Verification items for this drawing (mm, ordinates from the low corner). A direction names the side the tool comes from. Give positions to 0.01 mm unless a question says otherwise; leave off trailing zeros. Write each loop counter-clockwise with the first axis right and the second up, starting at its lowest first coordinate (ties: lowest second). Pieces come first, ordered by that corner, then holes. Notation, with made-up numbers: (36.25, -16.75) -> (65.25, -16.75) arc R21 ccw to (65.25, -11.75) -> close; hole circle Ø5 at (61, 25.5). An arc over 180 degrees is marked (long way). Answer as a JSON object with one key per item and string values.
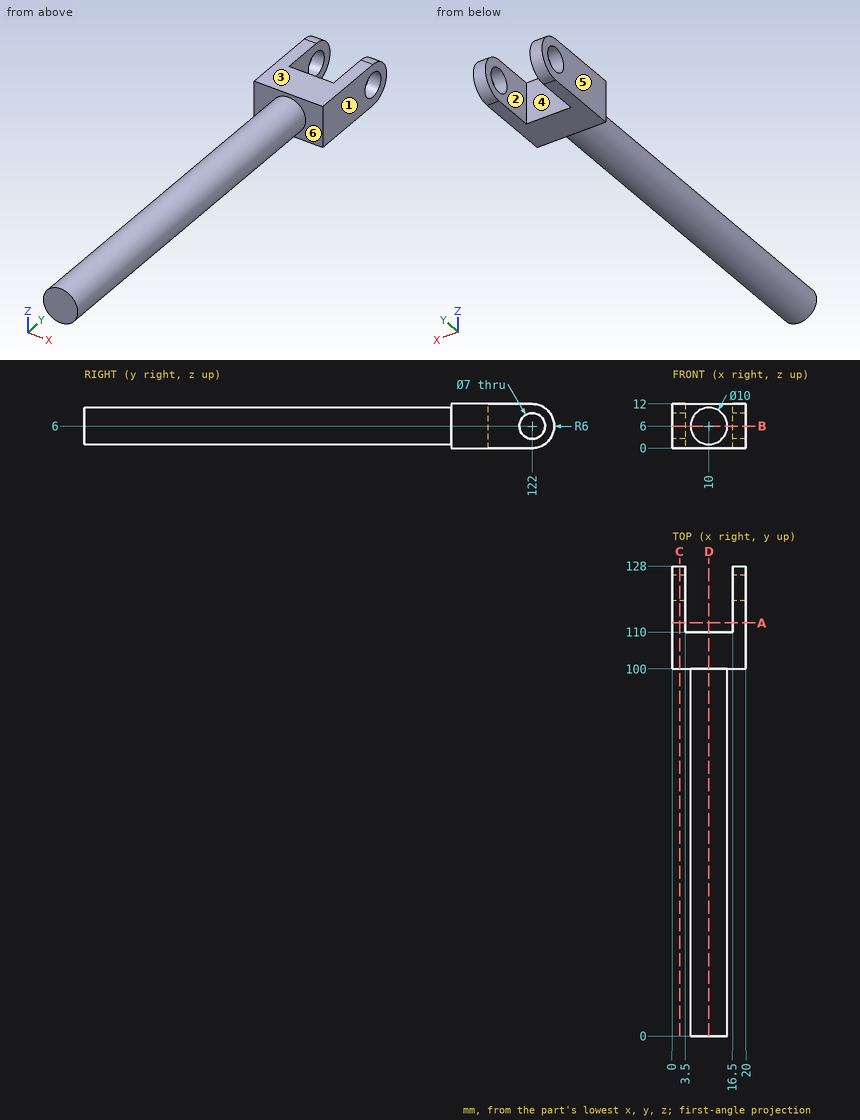
1. Sectioned sample at D-D, the plane x = 10. Enter the section's corners in (y, z).
Determined:
{"outline": "(0, 1) -> (100, 1) -> (100, 0) -> (110, 0) -> (110, 12) -> (100, 12) -> (100, 11) -> (0, 11) -> close"}
2. Scan lines: L1, parallel to Z at x = 18.6, y = 122; L2, parallel to Y at x = 1.85, z = 6; L3, parallel to X at y = 8, z = 6.25. Record each from-to range of solid material in increasing order. Write a range as [from, to].
Determined:
{"L1": "[0, 2.5], [9.5, 12]", "L2": "[100, 118.5], [125.5, 128]", "L3": "[5.01, 14.99]"}
3. Access from +Z, -Z, +X, -X, +Y, -Y to the whole of each face (thin tool, end or side, straight path). Record for the marked faces 4, 5 and 6.
Determined:
{"face 4": "+Z, -Z, +Y", "face 5": "+Z, -Z, -X, +Y, -Y", "face 6": "-Y"}
4. Sectioned sample at C-C, the plane x = 2. Enter the section's corners in (y, z).
Determined:
{"outline": "(100, 0) -> (122, 0) arc R6 ccw to (122, 12) -> (100, 12) -> close; hole circle Ø7 at (122, 6)"}
5. Sectioned sample at B-B, the plane z = 6. Enter the section's corners in (x, y), plus the area to 3 significant figures.
Determined:
{"outline": "(0, 100) -> (5, 100) -> (5, 0) -> (15, 0) -> (15, 100) -> (20, 100) -> (20, 118.5) -> (16.5, 118.5) -> (16.5, 110) -> (3.5, 110) -> (3.5, 118.5) -> (0, 118.5) -> close; (0, 125.5) -> (3.5, 125.5) -> (3.5, 128) -> (0, 128) -> close; (16.5, 125.5) -> (20, 125.5) -> (20, 128) -> (16.5, 128) -> close", "area": "1,280 mm^2"}
6. Sectioned sample at A-A, the plane y = 112.5. Enter the section's corners in (x, z), plus the area to 3 significant figures.
Determined:
{"outline": "(0, 0) -> (3.5, 0) -> (3.5, 12) -> (0, 12) -> close; (16.5, 0) -> (20, 0) -> (20, 12) -> (16.5, 12) -> close", "area": "84.0 mm^2"}
7. Mould release check, pull along X, two halves, no side actions. Record for the marked faces 1, 2 and 3: released by +X, released by -X, zero draft, split by the parting line, or undercut.
Determined:
{"face 1": "released by +X", "face 2": "undercut", "face 3": "zero draft"}
8. Go/stop test with flat-tipped pins: P1, Ø3.5, axis at x = 7.5, z = 3.5, coming from the +Y side; P2, Ø2, axis at x = 6.5, y = 80, coming from the -Z side; P3, Ø5, axis at y = 105, z = 9.5, coming from the -X side; P4, Ø12, axis at x = 6, y = 42.5, coming from the -Z side. Record where each tip stops, or that it passes through.
Determined:
{"P1": "y = 110", "P2": "z = 1.67", "P3": "x = 0", "P4": "z = 1"}
